Design review of the part built by this model. Coordinates are the model's own, in mm. A direction names the side the tool comes from. Coordinates: 2 decimals unless noted, no trailing zeros. Loops run counter-clockwise (first coordinate to the right, second up) from the corner with the lowest first, then second, coordinate; pieces in that order, holes last. Notation, with made-up numbers: (70, -5) -> (94, -5) arc R31 cw to (94, 27) -> close; hole circle Ø8 at (59, 79.25). An arc over 180 degrees is marked (long way). Answer in a Markdown table with one row per item.
```python
from build123d import *

# Parameters (mm, degrees)
BOSS_EXTRUDE1_DEPTH = 7.62
SKETCH2_R           = 2.159
CUT_EXTRUDE1_DEPTH  = 38.309477646
SKETCH3_R           = 1.5
CUT_EXTRUDE2_DEPTH  = 38.309477646


with BuildPart() as part:
    # Sketch1 → Boss-Extrude1 (new body)
    with BuildSketch(Plane.XY):
        Polygon((-8.747635235, -17.04359987), (-8.747635235, -19.58359987), (3.952364765, -19.58359987), (3.952364765, 18.41640013), (-8.747635235, 18.41640013), (-8.747635235, 15.87640013), (-1.127635235, 15.87640013), (-1.127635235, -17.04359987), align=None)
    extrude(amount=BOSS_EXTRUDE1_DEPTH)

    # Sketch2 → Cut-Extrude1 (cut, through all)
    with BuildSketch(Plane(origin=(0, -17.04359987, 0), x_dir=(1, 0, 0), z_dir=(0, 1, 0))):
        with Locations(Location((-4.937635235, -3.81, 0), (0, 0, 270))):
            Circle(SKETCH2_R)
    extrude(amount=-CUT_EXTRUDE1_DEPTH, mode=Mode.SUBTRACT)

    # Sketch3 → Cut-Extrude2 (cut, through all)
    with BuildSketch(Plane.XZ.offset(-15.87640013)):
        with Locations(Location((-4.937635235, 3.81, 0), (0, 0, 270))):
            Circle(SKETCH3_R)
    extrude(amount=-CUT_EXTRUDE2_DEPTH, mode=Mode.SUBTRACT)


solid = part.part
```
(1) Take a section at D-D on y = 16.5. Give the boundary of the cut face in (x, z), and give its area (3 significant figures).
Evaluation:
| item | result |
|---|---|
| outline | (-8.75, 0) -> (3.95, 0) -> (3.95, 7.62) -> (-8.75, 7.62) -> close; hole circle Ø3 at (-4.94, 3.81) |
| area | 89.7 mm² |
(2) For pin 1 (4 mm diameter, centred on y = -8, z = 5, fed in from -X), flat-tipped, find the tip position at first contact; note if it passes through.
Evaluation:
| item | result |
|---|---|
| pin 1 | stops at x = -1.13 |
(3) Take a section at A-A on z = 3.81. Give the boundary of the cut face in (x, y), and give its area (3 significant figures).
Evaluation:
| item | result |
|---|---|
| outline | (-8.75, -19.58) -> (-7.1, -19.58) -> (-7.1, -17.04) -> (-8.75, -17.04) -> close; (-8.75, 15.88) -> (-6.44, 15.88) -> (-6.44, 18.42) -> (-8.75, 18.42) -> close; (-3.44, 15.88) -> (-1.13, 15.88) -> (-1.13, -17.04) -> (-2.78, -17.04) -> (-2.78, -19.58) -> (3.95, -19.58) -> (3.95, 18.42) -> (-3.44, 18.42) -> close |
| area | 213 mm² |
(4) Take a section at B-B on x = -4.25. Give the boundary of the cut face in (y, z), and give its area (3 significant figures).
Evaluation:
| item | result |
|---|---|
| outline | (-19.58, 0) -> (-17.04, 0) -> (-17.04, 1.76) -> (-19.58, 1.76) -> close; (-19.58, 5.86) -> (-17.04, 5.86) -> (-17.04, 7.62) -> (-19.58, 7.62) -> close; (15.88, 0) -> (18.42, 0) -> (18.42, 2.48) -> (15.88, 2.48) -> close; (15.88, 5.14) -> (18.42, 5.14) -> (18.42, 7.62) -> (15.88, 7.62) -> close |
| area | 21.5 mm² |
(5) Take a section at C-C on z = 7.25. Give the boundary of the cut face in (x, y), and give its area (3 significant figures).
Evaluation:
| item | result |
|---|---|
| outline | (-8.75, -19.58) -> (3.95, -19.58) -> (3.95, 18.42) -> (-8.75, 18.42) -> (-8.75, 15.88) -> (-1.13, 15.88) -> (-1.13, -17.04) -> (-8.75, -17.04) -> close |
| area | 232 mm² |
(6) To check wall thickness, follow probe 1 along X at (y, z) = (17.9, 3.81); probe 2 along X at (y, z) = (-17.65, 3.81); probe 3 along Y at (x, z) = (-5, 0.5). State the ranges of each line that lie inside material, in increasing order.
Evaluation:
| item | result |
|---|---|
| probe 1 | x = -8.75 to -6.44, -3.44 to 3.95 |
| probe 2 | x = -8.75 to -7.1, -2.78 to 3.95 |
| probe 3 | y = -19.58 to -17.04, 15.88 to 18.42 |
(7) Draft analysis for pull direction Y (two halves, no side actions). For faces 4 (the flat face through (-8.748, 17, 4)), 5 (the flat face through (-2, 18.416, 4)), 6 (the flat face through (-7, 15.876, 4)), state which applies: pulls with the +Y half, pulls with the -Y half, needs draft (parallel to the pull), parting line crosses it, or undercut.
Evaluation:
| item | result |
|---|---|
| face 4 | needs draft |
| face 5 | pulls with the +Y half |
| face 6 | undercut |
(8) Tool access review of faces 1 (the cylindrical face through (-4.843, -18.296, 1.653)), 2 (the flat face through (-3, -17.044, 2)), 3 (the flat face through (-8.748, -18, 4)): name each direction out of +Z, -Z, +X, -X, +Y, -Y from which nothing blocks a thin tool from reaching the whole face with its end or side.
Evaluation:
| item | result |
|---|---|
| face 1 | -Y |
| face 2 | +Z, -Z, -X |
| face 3 | +Z, -Z, -X, +Y, -Y |
